Work out the finished part from the listing and answer in its coordinate system (mm). A direction names the side the tool comes from. Round coordinates to 2 decimals unless told otherwise and drop trailing zeros. Write each loop counter-clockwise with the first axis right and the second up, starting at its lowest first coordinate (ties: lowest second). Pieces come first, ordered by that corner, then holes. Notation, with made-up numbers: (-23.75, 42) -> (21.25, 42) arc R12 cw to (21.25, 61) -> close; hole circle Ø4 at (73, 84). An arc over 180 degrees is marked (long way). One line per item, written item: value.
```python
from build123d import *

# Parameters (mm, degrees)
F1_DEPTH  = 25
F2_W      = 25.5589389365
F2_H      = 4.2958939448
F3_DEPTH  = 1.7
F4_W      = 4.2958939448
F4_H      = 20.1124101877
F5_DEPTH  = 1.9
F6_W      = 4.4450499117
F6_H      = 20.1124101877
F8_DEPTH  = 1.8
F7_W      = 25.5589389365
F7_H      = 4.2430022731
F9_DEPTH  = 1.9
F11_DEPTH = 9.1


with BuildPart() as f1:
    # F0 (on Front) → F1 (new body)
    with BuildSketch(Plane.XZ):
        Polygon((-19.4574361484, 2.6685861076), (-44.104386121, 9.4352113083), (-47.3371483386, 3.9799264632), (-22.0899792911, 0), (-22.0899792911, -20.1124101877), (-15.6050544099, -20.1124101877), (-15.6050544099, 0), (9.6421146375, 3.9799264632), (5.3972699679, 8.6270207539), align=None)
    extrude(amount=F1_DEPTH)

    # F2 (on face) → F3 (cut)
    with BuildSketch(Plane(origin=(-0.378381367, 0, 2.4003102636), x_dir=(0.9878019236, 0, 0.1557156372), z_dir=(0.1557156372, 0, -0.9878019236))):
        with Locations((-2.6352332962, 12.8331626765)):
            Rectangle(F2_W, F2_H)
    extrude(amount=-F3_DEPTH, mode=Mode.SUBTRACT)

    # F4 (on face) → F5 (cut)
    with BuildSketch(Plane.YZ.offset(-15.6050544099)):
        with Locations((-12.8331626765, -10.0562050939)):
            Rectangle(F4_W, F4_H)
    extrude(amount=-F5_DEPTH, mode=Mode.SUBTRACT)

    # F6 (on face) → F8 (cut)
    with BuildSketch(Plane(origin=(-22.0899792911, 0, 0), x_dir=(0, -1, 0), z_dir=(-1, 0, 0))):
        with Locations((12.4689359218, -10.0562050939)):
            Rectangle(F6_W, F6_H)
    extrude(amount=-F8_DEPTH, mode=Mode.SUBTRACT)

    # F7 (on face) → F9 (cut)
    with BuildSketch(Plane(origin=(-0.5356236731, 0, -3.3977968049), x_dir=(0.9878019236, 0, -0.1557156372), z_dir=(-0.1557156372, 0, -0.9878019236))):
        with Locations((-34.599993505, 12.1658644639)):
            Rectangle(F7_W, F7_H)
    extrude(amount=-F9_DEPTH, mode=Mode.SUBTRACT)

    # F10 (on face) → F11 (cut)
    with BuildSketch(Plane.XZ.offset(25)):
        Polygon((-22.0899792911, 1.9871564582), (-46.0743617449, 6.1108782943), (-47.3371483386, 3.9799264632), (-22.0899792911, 0), align=None)
        Polygon((9.6421146375, 3.9799264632), (7.7104689044, 6.0946186502), (-15.6050544099, 2.4822140113), (-15.6050544099, 0), align=None)
    extrude(amount=-F11_DEPTH, mode=Mode.SUBTRACT)


solid = f1.part
```
(1) Find section B-B on z = -5.25. Give the vertices of the cut face in (x, y), plus the area to 3 significant figures.
Reported:
outline: (-22.09, -25) -> (-15.61, -25) -> (-15.61, -14.98) -> (-17.51, -14.98) -> (-17.51, -10.69) -> (-15.61, -10.69) -> (-15.61, 0) -> (-22.09, 0) -> (-22.09, -10.25) -> (-20.29, -10.25) -> (-20.29, -14.69) -> (-22.09, -14.69) -> close
area: 146 mm2
(2) Find section C-C on x = -21. Give the vertices of the cut face in (y, z).
Reported:
outline: (-25, -20.11) -> (-14.69, -20.11) -> (-14.69, 0) -> (-10.25, 0) -> (-10.25, -20.11) -> (0, -20.11) -> (0, 3.09) -> (-25, 3.09) -> close
(3) Find section D-D on y = -8.25. Give the vertices of the cut face in (x, z).
Reported:
outline: (-47.34, 3.98) -> (-22.09, 0) -> (-22.09, -20.11) -> (-15.61, -20.11) -> (-15.61, 0) -> (9.64, 3.98) -> (5.4, 8.63) -> (-19.46, 2.67) -> (-44.1, 9.44) -> close
(4) A tool of negligible diameter and unlimited length cuts with its end or side. For faces 1 (the face through (-3.784, -20.514, 4.314)), 2 (the face through (-17.505, -13, -10)), 3 (the face through (-22.09, -5, -10)), 4 (the face through (-15.605, -5, -10)), from which of +Z, -Z, +X, -X, +Y, -Y can it reach the whole face along a straight path? Write none if from no direction.
Reported:
face 1: -Z, +X, -Y
face 2: -Z, +X
face 3: -Z, -X, +Y, -Y
face 4: -Z, +X, +Y, -Y
(5) Find section A-A on y = -23. Give the vertices of the cut face in (x, z).
Reported:
outline: (-46.07, 6.11) -> (-22.09, 1.99) -> (-22.09, -20.11) -> (-15.61, -20.11) -> (-15.61, 2.48) -> (7.71, 6.09) -> (5.4, 8.63) -> (-19.46, 2.67) -> (-44.1, 9.44) -> close
(6) Consider probe 1 along Y at (x, z) = (-3, 2.5); probe 2 along X at (y, z) = (-23.5, 1.25); probe 3 along X at (y, z) = (-13, -9). Determine where each line is inside the solid, lowest interval first.
Reported:
probe 1: y = -15.9 to -14.98, -10.69 to 0
probe 2: x = -22.09 to -15.61
probe 3: x = -20.29 to -17.51
(7) Flat-ended cylindrical pins translate along their axes: pin 1 Ø12 at (x, y) = (-41, -4.5) entering from -Z; pin 2 Ø2 at (x, z) = (-21.5, -14.5) entering from +Y; pin 3 Ø1.5 at (x, y) = (-13.5, -16) entering from +Z; pin 4 Ø5 at (y, z) = (-7, -10.5) entering from -X. Find the tip coordinate at first contact, or state that the pin passes through.
Reported:
pin 1: stops at z = 2.04
pin 2: stops at y = 0
pin 3: stops at z = 4.28
pin 4: stops at x = -22.09
